Design review of the part built by this model. Coordinates are the model's own, in mm. Face numbers are marked on the shaded views. A direction names the side the tool comes from. Coordinates: 2 decimals unless noted, no trailing zeros. Write each loop counter-clockwise with the first axis right and the second up, starting at its lowest first coordinate (ties: lowest second). Pieces come first, ordered by that corner, then holes. Notation, with made-up numbers: M 53.25,24.25 L 87.25,24.25 A10 ccw 87.25,40.25 Z; hole C -0.75,0.25 d2. An arc over 180 degrees is marked long. Write item = value, one per line.
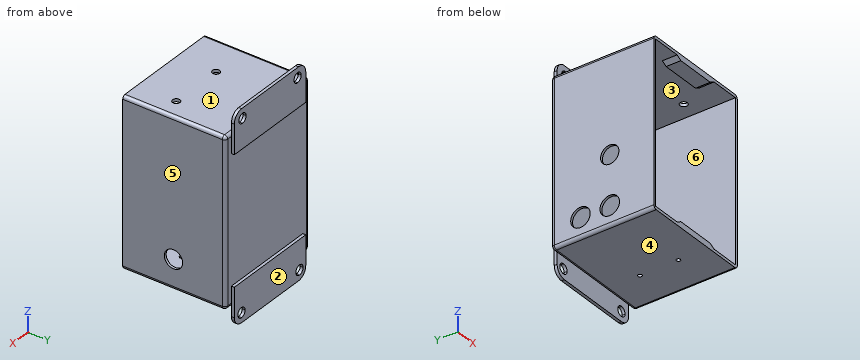
```python
from build123d import *

# Parameters (mm, degrees)
F1_DEPTH   = 66.802
F2_DEPTH   = 1.9
F3_DEPTH   = 1.9
F4_R       = 2.032
F5_DEPTH   = 12.7
F6_DEPTH   = 12.7
F7_R       = 6.35
F8_DEPTH   = 1.5875
F9_R       = 1.27
F10_DEPTH  = 3.81
F11_W      = 43.18
F11_H      = 55.3302187473
F1_FACE3_W = 18.7325
F1_FACE3_H = 64.902
F12_DEPTH  = 1.905
F13_W      = 43.18
F13_H      = 55.3302187473
F14_DEPTH  = 1.905
F15_R      = 2.3749
F16_DEPTH  = 1.905
F17_R      = 5.969
F18_DEPTH  = 1.5875
F19_R      = 5.969
F20_DEPTH  = 1.5875


with BuildPart() as f1:
    # F0 (on Front) → F1 (new body)
    with BuildSketch(Plane.XZ):
        Polygon((62.2927888, 122.2015844), (-0.2547112, 122.2015844), (-5.4934612, 122.2015844), (-5.4934612, 14.2515844), (-0.2547112, 14.2515844), (62.2927888, 14.2515844), (67.5315388, 14.2515844), (67.5315388, 122.2015844), align=None)
        Polygon((65.9440388, 120.2965844), (65.9440388, 16.1565844), (47.2115388, 16.1565844), (43.9119772, 18.0615844), (18.1261004, 18.0615844), (14.8265388, 16.1565844), (-3.9059612, 16.1565844), (-3.9059612, 120.2965844), (14.8265388, 120.2965844), (18.1261004, 118.3915844), (43.9119772, 118.3915844), (47.2115388, 120.2965844), align=None, mode=Mode.SUBTRACT)
    extrude(amount=F1_DEPTH)

    # F0 (on Front) → F3 (join)
    with BuildSketch(Plane.XZ):
        Polygon((47.2115388, 16.1565844), (65.9440388, 16.1565844), (65.9440388, 120.2965844), (47.2115388, 120.2965844), (43.9119772, 118.3915844), (18.1261004, 118.3915844), (14.8265388, 120.2965844), (-3.9059612, 120.2965844), (-3.9059612, 16.1565844), (14.8265388, 16.1565844), (18.1261004, 18.0615844), (43.9119772, 18.0615844), align=None)
    extrude(amount=F3_DEPTH)

    # F4
    f4_edges = [f1.edges().sort_by_distance(p)[0] for p in [
        (-5.493461, -33.401, 122.201584),
        (67.531539, -33.401, 122.201584),
        (67.531539, -33.401, 14.251584),
        (-5.493461, -33.401, 14.251584),
        (-5.493461, 0, 68.226584),
        (67.531539, 0, 68.226584),
        (31.019039, 0, 122.201584),
        (31.019039, 0, 14.251584),
    ]]
    fillet(f4_edges, radius=F4_R)



with BuildPart() as f2:
    # F0 (on Front) → F2 (new body)
    with BuildSketch(Plane.XZ):
        with BuildLine():
            Line((62.2927888, 14.2515844), (-0.2547112, 14.2515844))
            Line((-0.2547112, 14.2515844), (-0.2547112, 7.9015844))
            ThreePointArc((-0.2547112, 7.9015844), (1.6051607395, 3.4114563395), (6.0952888, 1.5515844))
            Line((6.0952888, 1.5515844), (55.9427888, 1.5515844))
            ThreePointArc((55.9427888, 1.5515844), (60.4329168605, 3.4114563395), (62.2927888, 7.9015844))
            Line((62.2927888, 7.9015844), (62.2927888, 14.2515844))
        make_face()
        with BuildLine():
            ThreePointArc((5.2507388, 11.0765844), (7.4958028303, 10.1466484303), (8.4257388, 7.9015844))
            ThreePointArc((8.4257388, 7.9015844), (7.4958028303, 5.6565203697), (5.2507388, 4.7265844))
            ThreePointArc((5.2507388, 4.7265844), (3.0056747697, 5.6565203697), (2.0757388, 7.9015844))
            ThreePointArc((2.0757388, 7.9015844), (3.0056747697, 10.1466484303), (5.2507388, 11.0765844))
        make_face(mode=Mode.SUBTRACT)
        with BuildLine():
            ThreePointArc((56.0253388, 11.0765844), (58.2704028303, 10.1466484303), (59.2003388, 7.9015844))
            ThreePointArc((59.2003388, 7.9015844), (58.2704028303, 5.6565203697), (56.0253388, 4.7265844))
            ThreePointArc((56.0253388, 4.7265844), (53.7802747697, 5.6565203697), (52.8503388, 7.9015844))
            ThreePointArc((52.8503388, 7.9015844), (53.7802747697, 10.1466484303), (56.0253388, 11.0765844))
        make_face(mode=Mode.SUBTRACT)
    extrude(amount=-F2_DEPTH)


with BuildPart() as f2b:
    # F0 (on Front) → F2, piece 2 (new body)
    with BuildSketch(Plane.XZ):
        with BuildLine():
            Line((55.9427888, 134.9015844), (6.0952888, 134.9015844))
            ThreePointArc((6.0952888, 134.9015844), (1.6051607395, 133.0417124605), (-0.2547112, 128.5515844))
            Line((-0.2547112, 128.5515844), (-0.2547112, 122.2015844))
            Line((-0.2547112, 122.2015844), (62.2927888, 122.2015844))
            Line((62.2927888, 122.2015844), (62.2927888, 128.5515844))
            ThreePointArc((62.2927888, 128.5515844), (60.4329168605, 133.0417124605), (55.9427888, 134.9015844))
        make_face()
        with BuildLine():
            ThreePointArc((6.8890388, 131.7265844), (9.1341028303, 130.7966484303), (10.0640388, 128.5515844))
            ThreePointArc((10.0640388, 128.5515844), (9.1341028303, 126.3065203697), (6.8890388, 125.3765844))
            ThreePointArc((6.8890388, 125.3765844), (4.6439747697, 126.3065203697), (3.7140388, 128.5515844))
            ThreePointArc((3.7140388, 128.5515844), (4.6439747697, 130.7966484303), (6.8890388, 131.7265844))
        make_face(mode=Mode.SUBTRACT)
        with BuildLine():
            ThreePointArc((55.1490388, 131.7265844), (57.3941028303, 130.7966484303), (58.3240388, 128.5515844))
            ThreePointArc((58.3240388, 128.5515844), (57.3941028303, 126.3065203697), (55.1490388, 125.3765844))
            ThreePointArc((55.1490388, 125.3765844), (52.9039747697, 126.3065203697), (51.9740388, 128.5515844))
            ThreePointArc((51.9740388, 128.5515844), (52.9039747697, 130.7966484303), (55.1490388, 131.7265844))
        make_face(mode=Mode.SUBTRACT)
    extrude(amount=-F2_DEPTH)


with BuildPart() as f1_1:
    add(f1.part)
    # F5 (add): a face of the model
    f5_faces = [f2.part.faces().sort_by_distance(p)[0] for p in [
        (31.0190388, 0.95, 14.2515844),
    ]]

    add(f2.part)  # F5 merges F2
    extrude(f5_faces, amount=F5_DEPTH)

    # F6 (add): a face of the model
    f6_faces = [f2b.part.faces().sort_by_distance(p)[0] for p in [
        (31.0190388, 0.95, 122.2015844),
    ]]

    add(f2b.part)  # F6 merges F2b
    extrude(f6_faces, amount=F6_DEPTH)

    # F7 (on face) → F8 (cut, through all)
    with BuildSketch(Plane(origin=(-5.4934612, 0, 0), x_dir=(0, -1, 0), z_dir=(-1, 0, 0))):
        with Locations((38.1, 26.9515844)):
            Circle(F7_R)
        with Locations((19.05, 26.9515844)):
            Circle(F7_R)
    extrude(amount=-F8_DEPTH, mode=Mode.SUBTRACT)

    # F9 (on face) → F10 (cut, through all)
    with BuildSketch(Plane(origin=(0, 0, 14.2515844), x_dir=(1, 0, 0), z_dir=(0, 0, -1))):
        with Locations((42.1315388, 47.352)):
            Circle(F9_R)
        with Locations((42.1315388, 22.352)):
            Circle(F9_R)
    extrude(amount=-F10_DEPTH, mode=Mode.SUBTRACT)

    # F11 (on face) + F1_face3 (on face) → F12 (cut, through all)
    with BuildSketch(Plane(origin=(0, 0, 118.3915844), x_dir=(1, 0, 0), z_dir=(0, 0, -1))):
        with Locations((32.6428469086, 29.5651093736)):
            Rectangle(F11_W, F11_H)
    with BuildSketch(Plane(origin=(5.4602888, -34.351, 16.1565844), x_dir=(1, 0, 0), z_dir=(0, 0, 1))):
        Rectangle(F1_FACE3_W, F1_FACE3_H)
    extrude(amount=-F12_DEPTH, dir=(0, 0, -1), mode=Mode.SUBTRACT)

    # F13 (on face) → F14 (cut, through all)
    with BuildSketch(Plane.XY.offset(18.0615844)):
        with Locations((30.3840388, -29.5651093736)):
            Rectangle(F13_W, F13_H)
    extrude(amount=-F14_DEPTH, mode=Mode.SUBTRACT)

    # F15 (on face) → F16 (cut, through all)
    with BuildSketch(Plane.XY.offset(122.2015844)):
        with Locations((19.9065388, -41.402)):
            Circle(F15_R)
        with Locations((54.8315388, -41.402)):
            Circle(F15_R)
    extrude(amount=-F16_DEPTH, mode=Mode.SUBTRACT)

    # F17 (on face) → F18 (cut, through all)
    with BuildSketch(Plane.YZ.offset(67.5315388)):
        with Locations((-33.782, 33.3015844)):
            Circle(F17_R)
    extrude(amount=-F18_DEPTH, mode=Mode.SUBTRACT)

    # F19 (on face) → F20 (cut, through all)
    with BuildSketch(Plane(origin=(-5.4934612, 0, 0), x_dir=(0, -1, 0), z_dir=(-1, 0, 0))):
        with Locations((38.1, 58.7015844)):
            Circle(F19_R)
    extrude(amount=-F20_DEPTH, mode=Mode.SUBTRACT)


solid = f1_1.part
```
Q1. The part is to be moulded in two halves that separate along Z. For the marked faces 1, 2 and 3, say which applies: +Z half, -Z half, draft (parallel to the pull), parting line (faces both ways), or undercut.
Check result:
face_1 = +Z half
face_2 = draft
face_3 = undercut
Q2. For P1, Ø12, axis at x = 41, y = -9.5, coming from the -Z side; P2, Ø2, axis at x = 51, y = -38.5, coming from the +Z side; P3, Ø7.5, axis at x = 46, z = 6, coming from the -Y side, all flat-tipped, find the tip position at first contact; note any pin that passes through.
Check result:
P1 = 14.25
P2 = 122.2
P3 = 0
Q3. Wall thickness on line 1 (X direction, y = -6, z = 62.5); line 2 (Z direction, x = 63, y = -39); line 3 (Z direction, x = -4.3, y = -38.1): over which ranges is each line inside the solid? List them lowest first.
Check result:
line_1 = -5.49 to -3.91, 65.94 to 67.53
line_2 = 14.25 to 16.16, 120.3 to 122.2
line_3 = 14.43 to 20.6, 33.3 to 52.73, 64.67 to 122.02
Q4. Consider section B-B, the plane y = -19.05. State the section outline as (x, z) points, and give its area (3 significant figures).
Check result:
outline = M -5.49,16.28 A2.03 ccw -3.46,14.25 L 65.5,14.25 A2.03 ccw 67.53,16.28 L 67.53,120.17 A2.03 ccw 65.5,122.2 L -3.46,122.2 A2.03 ccw -5.49,120.17 L -5.49,33.3 L -3.91,33.3 L -3.91,120.3 L 65.94,120.3 L 65.94,16.16 L -3.91,16.16 L -3.91,20.6 L -5.49,20.6 Z
area = 585 mm²
Q5. Machinability: for the marked faces 4, 5 and 6, which of the approach directions +Z, -Z, +X, -X, +Y, -Y give a long, thin tool a straight path to every point of the face, cutting with its end or side? Answer none if there is none.
Check result:
face_4 = -Z, +X, -X, -Y
face_5 = +Z, -Z, +X, +Y, -Y
face_6 = -Y
Q6. Consider section A-A, the plane z = 95. State the section outline as (x, y) points, and give its area (3 significant figures).
Check result:
outline = M -5.49,-66.8 L -3.91,-66.8 L -3.91,-1.9 L 65.94,-1.9 L 65.94,-66.8 L 67.53,-66.8 L 67.53,-2.03 A2.03 ccw 65.5,0 L -3.46,0 A2.03 ccw -5.49,-2.03 Z
area = 343 mm²
